Input: part model. Units: mm. Frame: model coordinates. A direction names the side the tool comes from. Coordinates: 2 decimals unless noted, no trailing zeros. Loops run counter-clockwise (first coordinate to the right, second up) from the corner with the lowest first, then second, coordinate; pieces in that order, holes last.
(1) Line query: L1, parallel to Y at x = 139.7, z = -1.4; L2, parallel to Z at x = 12.7, y = 0.8; L3, parallel to Y at x = 109.5, z = -21. Output: solid intervals per line, ascending.
(2) Mould query, pull axis Y, two halves, no side actions, for faces 3 (the face through (150, 0, -13)), 4 (the face through (168.03, 1.6, -17.17)), 5 (the face through (166.565, 13.134, -1.603)). Classes: released by +Y, released by -Y, zero draft, split by the parting line, or undercut.
(3) Set-up query: faces 1 (the face through (150, 14, -3.251)), 2 (the face through (0, 7, -3)). Return all of +Z, -Z, +X, -X, +Y, -Y with unobstructed straight access to the full face (end or side cutting, diameter ignored); none if empty.
(4) Section A-A, the plane x = 165.1. Return loops of the section in (y, z), then the cut area to 3 significant figures.
(5) Section B-B, the plane x = 72. Return loops of the section in (y, z).
(6) Contact query for flat-ended pins moving along their axis: P1, Ø4, axis at x = 263, y = 4.5, coming from the -Z side; P2, Ø1.5, axis at x = 236.5, z = -20, coming from the +Y side. Output: stop coordinate, or through.
Autodesk Inventor part; units mm, degrees
ref_plane "YZ Plane" through (0, 0, 0) normal (1, 0, 0) x (0, 1, 0)
ref_plane "XZ Plane" through (0, 0, 0) normal (0, 1, 0) x (-1, 0, 0)
ref_plane "XY Plane" through (0, 0, 0) normal (0, 0, 1) x (1, 0, 0)
sketch "Sketch1" plane through (0, 0, 0) normal (1, 0, 0) x (0, 1, 0)
  line L0 (0, 0) -> (25.4, 0)
  line L1 (3.2512, -25.4) -> (0, -25.4)
  line L2 (0, -25.4) -> (0, 0)
  line L3 (3.2512, -3.2512) -> (25.4, -3.2512)
  line L4 (3.2512, -25.4) -> (3.2512, -3.2512)
  line L5 (25.4, 0) -> (25.4, -3.2512)
  dimension "d0" = 25.4
  dimension "d1" = 3.2512
extrude "Extrusion1" add sketch "Sketch1" along normal blind 304.8
sketch "Sketch2" plane through (0, 0, -25.4) normal (0, -1, 0) x (1, 0, 0)
  line L0 (0, 9.4488) -> (110.0411, 9.4488) construction
  line L1 (0, 25.4) -> (304.8, 25.4)
  circle A0 centre (12.7, 9.4488) radius 3.175
  circle A1 centre (139.7, 9.4488) radius 3.175
  line L2 (0, 0) -> (0, 25.4)
  line L3 (0, 0) -> (304.8, 0)
  line L4 (152.4, 25.4) -> (152.4, 0)
  circle A2 centre (292.1, 9.4488) radius 3.175
  circle A3 centre (165.1, 9.4488) radius 3.175
  dimension "d4" = 15.9512
  dimension "d5" = 6.35
  dimension "d6" = 12.7
  dimension "d7" = 139.7
extrude "Extrusion2" cut sketch "Sketch2" against normal blind 304.8 contours A0 | A1 | A2 | A3
sketch "Sketch3" plane through (0, 0, 0) normal (0, 0, 1) x (1, 0, 0)
  line L0 (0, 0) -> (0, 25.4)
  line L1 (0, 15.9512) -> (148.4119, 15.9512) construction
  line L2 (0, 0) -> (304.8, 0)
  circle A0 centre (12.7, 15.9512) radius 3.175
  circle A1 centre (139.7, 15.9512) radius 3.175
  line L3 (152.4, 0) -> (152.4, 21.95) construction
  circle A2 centre (292.1, 15.9512) radius 3.175
  circle A3 centre (165.1, 15.9512) radius 3.175
  dimension "d10" = 15.9512
  dimension "d11" = 6.35
  dimension "d12" = 12.7
  dimension "d13" = 139.7
extrude "Extrusion3" cut sketch "Sketch3" against normal blind 304.8
properties part number "Middle short L"
Report:
1. L1: y = 0 to 12.78, 19.13 to 25.4
1. L2: z = -25.4 to -19.13, -12.78 to 0
1. L3: y = 0 to 3.25
2. face 3: released by -Y
2. face 4: zero draft
2. face 5: undercut
3. face 1: -Z, +X, -X, +Y
3. face 2: +Z, -Z, -X, +Y, -Y
4. outline: (0, -25.4) - (3.25, -25.4) - (3.25, -19.13) - (0, -19.13) - close; (0, -12.78) - (3.25, -12.78) - (3.25, -3.25) - (12.78, -3.25) - (12.78, 0) - (0, 0) - close; (19.13, -3.25) - (25.4, -3.25) - (25.4, 0) - (19.13, 0) - close
4. area: 113 mm2
5. outline: (0, -25.4) - (3.25, -25.4) - (3.25, -3.25) - (25.4, -3.25) - (25.4, 0) - (0, 0) - close
6. P1: stops at z = -25.4
6. P2: stops at y = 3.25
